Can you work these out from the model? Positions are in its coordinate system, mm. A direction names the side the tool comes from. Coordinates: 2 decimals unless noted, no trailing zeros. Loops run counter-clockwise (first coordinate to the right, second up) from the corner with the lowest first, then second, coordinate; pieces in that order, holes last. Notation, with made-up numbers: M -23.5,80 L 25.5,80 A19 cw 25.5,111 Z; hole C 18,86.5 d8. An arc over 180 degrees is marked long. Answer as a JSON object with one key per item and string values. Group by question number.
Item 1: Suppose I cut it at C-C (y = 93). Write out the boundary of the cut face in (x, z).
Item 2: Which directions (+Z, -Z, +X, -X, +Y, -Y) give clear straight access to the entire face, cutting with the end or side of a thin tool? Please do faces 1 (the flat face through (5, 14, 6)), 2 (the flat face through (2.4, 97, 7)), 3 (the flat face through (2.6, -52, 7)).
Item 3: If I drill on line 1 (Y direction, x = 1.35, z = 1.5); line 2 (Y direction, x = 3.65, z = 9.75); line 3 (Y direction, x = 2.35, z = 6.75), over which ranges is the centre line in solid material (lowest first)?
Item 4: I'm going to push flat-ended pins straight in: pin 1 Ø3.5 at (y, z) = (94, 5.5) entering from +X; pin 2 Ø1.9 at (x, y) = (1.5, 98.5) entering from -Z; pin 3 Ø0.7 at (x, z) = (3, 4) entering from +Y. Where does each tip first touch, or does it pass through?
Item 5: Suppose I cut it at B-B (z = 8.75). Write out the boundary of the cut face in (x, y).
Item 6: Suppose I cut it at A-A (x = 0.8). Write out the boundary of the cut face in (y, z).
```python
from build123d import *

# Parameters (mm, degrees)
F1_DEPTH = 5
F2_R     = 1.5
F3_W     = 2.6
F3_H     = 15
F4_DEPTH = 12.001


with BuildPart() as f1:
    # F0 (on Right) → F1 (new body)
    with BuildSketch(Plane.YZ):
        Polygon((-59.212235, 12), (-59.212235, 0), (-55.212235, 0), (-55.212235, 6), (-49.012235, 6), (-49.012235, 0), (94.587765, 0), (94.587765, 6), (100.787765, 6), (100.787765, 0), (104.787765, 0), (104.787765, 12), align=None)
    extrude(amount=F1_DEPTH)

    # F2
    f2_edges = [f1.edges().sort_by_distance(p)[0] for p in [
        (5, -55.212235, 3),
        (5, -49.012235, 3),
    ]]
    fillet(f2_edges, radius=F2_R)

    # F3 (on face) → F4 (cut, through all)
    with BuildSketch(Plane.XY.offset(12)):
        with Locations((3.7, 97.287765)):
            Rectangle(F3_W, F3_H)
        with Locations((1.3, -51.712235)):
            Rectangle(F3_W, F3_H)
    extrude(amount=-F4_DEPTH, mode=Mode.SUBTRACT)


solid = f1.part
```
From the geometry:
{
 "1": {"outline": "M 0,0 L 2.4,0 L 2.4,12 L 0,12 Z"},
 "2": {"face 1": "+Z, -Z, +X, +Y, -Y", "face 2": "+Z, -Z, +X, +Y", "face 3": "+Z, -Z, -X, -Y"},
 "3": {"line 1": "-44.21 to 94.59, 100.79 to 104.79", "line 2": "-59.21 to 89.79", "line 3": "-44.21 to 104.79"},
 "4": {"pin 1": "x = 2.4", "pin 2": "z = 6", "pin 3": "y = 89.79"},
 "5": {"outline": "M 0,-44.21 L 2.6,-44.21 L 2.6,-59.21 L 5,-59.21 L 5,89.79 L 2.4,89.79 L 2.4,104.79 L 0,104.79 Z"},
 "6": {"outline": "M -44.21,0 L 94.59,0 L 94.59,6 L 100.79,6 L 100.79,0 L 104.79,0 L 104.79,12 L -44.21,12 Z"}
}
